from build123d import *

# Parameters (mm, degrees)
SZKIC1_R                    = 5
DODANIE_WYCI_GNI_CIE1_DEPTH = 3


with BuildPart() as part:
    # Szkic1 → Dodanie-wyciągnięcie1 (new body)
    with BuildSketch(Plane(origin=(0, 0, -1.5), x_dir=(-1, 0, 0), z_dir=(0, 0, -1))):
        with BuildLine():
            Line((-12, 0), (-12, -28.217670017))
            Line((-12, -28.217670017), (-10.5, -28.217670017))
            ThreePointArc((-10.5, -28.217670017), (0, -22.5), (10.5, -28.217670017))
            Line((10.5, -28.217670017), (12, -28.217670017))
            Line((12, -28.217670017), (12, 0))
            ThreePointArc((12, 0), (0, 12), (-12, 0))
        make_face()
        Circle(SZKIC1_R, mode=Mode.SUBTRACT)
    extrude(amount=-DODANIE_WYCI_GNI_CIE1_DEPTH)


solid = part.part
Here's how the part is built. I have some questions about the finished solid (model axes, mm). Coordinates: 2 decimals unless noted, no trailing zeros. Loops run counter-clockwise (first coordinate to the right, second up) from the corner with the lowest first, then second, coordinate; pieces in that order, holes last.
1. For P1, Ø1, axis at x = 3, z = -0.5, coming from the +Y side; P2, Ø1, axis at x = -8, z = -0.5, coming from the +Y side, each with a flat end and sliding along its axis, tell me the tip position at first contact or that it passes through.
2. Imagine slicing it at A-A, the plane x = 0. Please give me the cut outline in (y, z).
3. Imagine slicing it at B-B, the plane z = 0.45. Please give me the cut outline in (x, y), and give its area (3 significant figures).
4. Imagine slicing it at C-C, the plane y = -0.5. Please give me the cut outline in (x, z).
5. I need wall thicknesses on L1, parallel to Y at x = 0, z = -0.9; L2, parallel to X at y = -3, z = -1.05; L3, parallel to X at y = -25, z = 1.2. Which ranges of each line are inside material? Lowest first, please.
6. Imagine slicing it at D-D, the plane x = 9.25. Please give me the cut outline in (y, z).
7. If we mould it in two halves opening along X, with no side actions, what happens to faces 1 (the flat face through (12, -14, 0)), 2 (the cylindrical face through (0.2, -22.5, 0)), 3 (the flat face through (11, -28.218, 0))? For each: pulls with the +X half, pulls with the -X half, needs draft (parallel to the pull), parting line crosses it, or undercut.
Taken from the geometry:
1. P1: stops at y = 11.74
1. P2: stops at y = 9.37
2. outline: (-22.5, -1.5) - (-5, -1.5) - (-5, 1.5) - (-22.5, 1.5) - close; (5, -1.5) - (12, -1.5) - (12, 1.5) - (5, 1.5) - close
3. outline: (-12, -28.22) - (-10.5, -28.22) arc R12.5 cw to (10.5, -28.22) - (12, -28.22) - (12, 0) arc R12 ccw to (-12, 0) - close; hole circle Ø10 at (0, 0)
3. area: 740 mm2
4. outline: (-12, -1.5) - (-4.97, -1.5) - (-4.97, 1.5) - (-12, 1.5) - close; (4.97, -1.5) - (12, -1.5) - (12, 1.5) - (4.97, 1.5) - close
5. L1: y = -22.5 to -5, 5 to 12
5. L2: x = -12 to -4, 4 to 12
5. L3: x = -12 to -7.5, 7.5 to 12
6. outline: (-26.59, -1.5) - (7.64, -1.5) - (7.64, 1.5) - (-26.59, 1.5) - close
7. face 1: pulls with the +X half
7. face 2: undercut
7. face 3: needs draft
